from build123d import *

# Parameters (mm, degrees)
BOSS_EXTRUDE1_DEPTH = 50
CUT_EXTRUDE1_DEPTH  = 71.356236397
CUT_EXTRUDE2_DEPTH  = 50


with BuildPart() as part:
    # Sketch1 → Boss-Extrude1 (new body)
    with BuildSketch(Plane.XY):
        Polygon((0, 0), (35, 0), (35, 5), (5, 5), (5, 35), (0, 35), align=None)
    extrude(amount=BOSS_EXTRUDE1_DEPTH)

    # Sketch3 → Cut-Extrude1 (cut, through all)
    with BuildSketch(Plane.ZY):
        with BuildLine():
            ThreePointArc((29.999165768, 17.5), (28.534944015, 21.034944015), (25, 22.499165768))
            Line((25, 22.499165768), (25, 12.500834232))
            ThreePointArc((25, 12.500834232), (28.534944015, 13.965055985), (29.999165768, 17.5))
        make_face()
        with BuildLine():
            Line((25, 12.500834232), (25, 22.499165768))
            ThreePointArc((25, 22.499165768), (20.000834232, 17.5), (25, 12.500834232))
        make_face()
    extrude(amount=-CUT_EXTRUDE1_DEPTH, mode=Mode.SUBTRACT)

    # Sketch2 → Cut-Extrude2 (cut)
    with BuildSketch(Plane(origin=(0, 5, 0), x_dir=(1, 0, 0), z_dir=(0, 1, 0))):
        with BuildLine():
            ThreePointArc((15, -25), (20, -30), (25, -25))
            Line((25, -25), (15, -25))
        make_face()
        with BuildLine():
            Line((15, -25), (25, -25))
            ThreePointArc((25, -25), (20, -20), (15, -25))
        make_face()
    extrude(amount=-CUT_EXTRUDE2_DEPTH, mode=Mode.SUBTRACT)


solid = part.part
Model file for the job. Use its own axes, mm. A direction names the side the tool comes from. Give positions to 0.01 mm unless a question says otherwise; leave off trailing zeros. Loops run counter-clockwise (first coordinate to the right, second up) from the corner with the lowest first, then second, coordinate; pieces in that order, holes last. Notation, with made-up numbers: (-22.75, 86.25) -> (23.25, 86.25) arc R13 cw to (23.25, 104.25) -> close; hole circle Ø3 at (41.5, -12). An arc over 180 degrees is marked (long way). Use a Markdown table: item, result. Add a question column.
(1) Mould opens along Z. For faces 3 (the flat face through (4, 11, 0)), 4 (the flat face through (4, 11, 50)), 5 (the cylindrical face through (18.92, 2.54, 29.88)) say: +Z half, -Z half, draft (parallel to the pull), parting line (faces both ways), or undercut.
(2) Tool access for faces 1 (the flat face through (3, 35, 25)), 2 (the flat face through (20, 5, 19)): list every direction of +Z, -Z, +X, -X, +Y, -Y with a clear straight run to the whole face (end or side of a thin tool).
(3) Slice it at C-C on z = 41.5. List the corners of the cut face in (x, y).
(4) Wall check: line 1 along X through (y, z) = (3, 25); line 2 along Z through (x, y) = (20, 3.2); line 3 along X through (y, z) = (20.5, 47). Give the ranges that are in metal, low to high.
(5) Slice it at D-D on y = 32.5. List the corners of the cut face in (x, z).
(6) Slice it at A-A on x = 23. List the corners of the cut face in (y, z), and give its area (3 significant figures).
(7) Drop flat-ended pins along their axis: pin 1 Ø15 at (x, z) = (13.5, 15.5) entering from +Y; pin 2 Ø12 at (y, z) = (18, 9) entering from -X; pin 3 Ø9 at (y, z) = (26.5, 12.5) entering from +X. Give the stop position or say it passes through.
Filled sheet:
| question | item | result |
|---|---|---|
| 1 | face 3 | -Z half |
| 1 | face 4 | +Z half |
| 1 | face 5 | undercut |
| 2 | face 1 | +Z, -Z, +X, -X, +Y |
| 2 | face 2 | +Z, -Z, +X, +Y |
| 3 | outline | (0, 0) -> (35, 0) -> (35, 5) -> (5, 5) -> (5, 35) -> (0, 35) -> close |
| 4 | line 1 | 0 to 15, 25 to 35 |
| 4 | line 2 | 0 to 20, 30 to 50 |
| 4 | line 3 | 0 to 5 |
| 5 | outline | (0, 0) -> (5, 0) -> (5, 50) -> (0, 50) -> close |
| 6 | outline | (0, 0) -> (5, 0) -> (5, 21) -> (0, 21) -> close; (0, 29) -> (5, 29) -> (5, 50) -> (0, 50) -> close |
| 6 | area | 210 mm2 |
| 7 | pin 1 | y = 5 |
| 7 | pin 2 | x = 0 |
| 7 | pin 3 | x = 5 |
